from build123d import *

# Parameters (mm, degrees)
SKETCH1_W                    = 381
SKETCH1_H                    = 149.225
BOSS_EXTRUDE1_DEPTH          = 6.35
F_1_4_CLEARANCE_HOLE1_D      = 6.7564
CUT_EXTRUDE1_DEPTH           = 410.23028129
F_1_2_0_5_DIAMETER_HOLE1_D   = 12.7
F_10_0_1935_DIAMETER_HOLE1_D = 4.9149
SKETCH9_W                    = 19.05
SKETCH9_H                    = 14.2875
CUT_EXTRUDE2_DEPTH           = 410.23028129
FILLET1_R                    = 3.175


with BuildPart() as part:
    # Sketch1 → Boss-Extrude1 (new body)
    with BuildSketch(Plane(origin=(0, 0, 0), x_dir=(1, 0, 0), z_dir=(0, 1, 0))):
        with Locations((190.5, 74.6125)):
            Rectangle(SKETCH1_W, SKETCH1_H)
        with BuildLine():
            Line((342.9, 95.25), (342.9, 53.975))
            ThreePointArc((342.9, 53.975), (341.97006403, 51.72993597), (339.725, 50.8))
            Line((339.725, 50.8), (257.175, 50.8))
            ThreePointArc((257.175, 50.8), (254.92993597, 51.72993597), (254, 53.975))
            Line((254, 53.975), (254, 95.25))
            ThreePointArc((254, 95.25), (254.92993597, 97.49506403), (257.175, 98.425))
            Line((257.175, 98.425), (339.725, 98.425))
            ThreePointArc((339.725, 98.425), (341.97006403, 97.49506403), (342.9, 95.25))
        make_face(mode=Mode.SUBTRACT)
        with BuildLine():
            Line((41.275, 98.425), (123.825, 98.425))
            ThreePointArc((123.825, 98.425), (126.07006403, 97.49506403), (127, 95.25))
            Line((127, 95.25), (127, 53.975))
            ThreePointArc((127, 53.975), (126.07006403, 51.72993597), (123.825, 50.8))
            Line((123.825, 50.8), (41.275, 50.8))
            ThreePointArc((41.275, 50.8), (39.02993597, 51.72993597), (38.1, 53.975))
            Line((38.1, 53.975), (38.1, 95.25))
            ThreePointArc((38.1, 95.25), (39.02993597, 97.49506403), (41.275, 98.425))
        make_face(mode=Mode.SUBTRACT)
    extrude(amount=BOSS_EXTRUDE1_DEPTH)

    # 1/4 Clearance Hole1 (through all)
    with Locations(Plane(origin=(0, 6.35, 0), x_dir=(1, 0, 0), z_dir=(0, 1, 0))):
        with Locations((154.94, 74.6125), (186.69, 74.6125), (194.31, 74.6125), (226.06, 74.6125)):
            Hole(F_1_4_CLEARANCE_HOLE1_D / 2)

    # Sketch4 → Cut-Extrude1 (cut, through all)
    with BuildSketch(Plane(origin=(0, 6.35, 0), x_dir=(1, 0, 0), z_dir=(0, 1, 0))):
        with BuildLine():
            Line((186.69, 77.9907), (194.31, 77.9907))
            ThreePointArc((194.31, 77.9907), (197.6882, 74.6125), (194.31, 71.2343))
            Line((194.31, 71.2343), (186.69, 71.2343))
            ThreePointArc((186.69, 71.2343), (183.3118, 74.6125), (186.69, 77.9907))
        make_face()
    extrude(amount=-CUT_EXTRUDE1_DEPTH, mode=Mode.SUBTRACT)

    # 1/2 (0.5) Diameter Hole1 (through all)
    with Locations(Plane(origin=(19.05, 6.35, -130.175), x_dir=(0, 0, 1), z_dir=(0, 1, 0))):
        with Locations((0, 0), (111.125, 0), (0, 342.9), (111.125, 342.9)):
            Hole(F_1_2_0_5_DIAMETER_HOLE1_D / 2)

    # #10 (0.1935) Diameter Hole1 (through all)
    with Locations(Plane(origin=(0, 6.35, 0), x_dir=(1, 0, 0), z_dir=(0, 1, 0))):
        with Locations((19.05, 74.6125), (361.95, 74.6125)):
            Hole(F_10_0_1935_DIAMETER_HOLE1_D / 2)

    # Sketch9 → Cut-Extrude2 (cut, through all)
    with BuildSketch(Plane(origin=(0, 6.35, 0), x_dir=(1, 0, 0), z_dir=(0, 1, 0))):
        with Locations((117.475, 102.39375)):
            Rectangle(SKETCH9_W, SKETCH9_H)
        with Locations((117.475, 46.83125)):
            Rectangle(SKETCH9_W, SKETCH9_H)
        with Locations((263.525, 46.83125)):
            Rectangle(SKETCH9_W, SKETCH9_H)
        with Locations((263.525, 102.39375)):
            Rectangle(SKETCH9_W, SKETCH9_H)
    extrude(amount=-CUT_EXTRUDE2_DEPTH, mode=Mode.SUBTRACT)

    # Fillet1
    fillet1_edges = [part.edges().sort_by_distance(p)[0] for p in [
        (273.05, 3.175, -50.8),
        (273.05, 3.175, -98.425),
        (107.95, 3.175, -98.425),
        (107.95, 3.175, -50.8),
        (273.05, 3.175, -109.5375),
        (254, 3.175, -109.5375),
        (273.05, 3.175, -39.6875),
        (254, 3.175, -39.6875),
        (107.95, 3.175, -39.6875),
        (127, 3.175, -39.6875),
        (107.95, 3.175, -109.5375),
        (127, 3.175, -109.5375),
    ]]
    fillet(fillet1_edges, radius=FILLET1_R)


solid = part.part
The listing builds one solid part. Answer for the finished solid, in the listing's coordinates (mm). A direction names the side the tool comes from. Coordinates: 2 decimals unless noted, no trailing zeros. Loops run counter-clockwise (first coordinate to the right, second up) from the corner with the lowest first, then second, coordinate; pieces in that order, holes last. Notation, with made-up numbers: (9.5, -3) -> (41.5, -3) arc R11 cw to (41.5, 7) -> close; hole circle Ø2 at (33, 7). An arc over 180 degrees is marked (long way). Answer in a Markdown table with one row per item. Add a question column.
1. Consider line 1 (X direction, y = 4.5, z = -85.5); line 2 (Z direction, x = 361.95, y = 4.5) (3 decimals); line 3 (X direction, y = 3.5, z = -130). Determine where each line is inside the solid, lowest interval first. Write a range as [from, to].
2. A flat-ended cylindrical pin translates along its axis: P1, Ø1.9, axis at x = 190, y = 2.5, coming from the +Z side. Find the tip coordinate at first contact, or state that the pin passes through.
3. The part is cut by section C-C, the plane x = 68. Write down the section's boundary in (y, z) (3 decimals), then the cut area to 3 significant figures.
4. For faces 4 (the flat face through (73, 3, -98.425)), 5 (the flat face through (188, 3, 0)), determine the directions among +Z, -Z, +X, -X, +Y, -Y from which every point of the face is accessible in a straight line to the end or side of a thin tool.
5. The part is cut by section B-B, the plane x = 226.06. Write down the section's boundary in (y, z) (3 decimals), then the cut area to 3 significant figures.
6. The part is cut by section A-A, the plane z = -82.5. Write down the section's boundary in (x, y), then the cut area to 3 significant figures.
7. The part is cut by section D-D, the plane z = -129. Write down the section's boundary in (x, y), then the cut area to 3 significant figures.
8. Determine the mould class of faces 1 (the flat face through (73, 3, -50.8)), 2 (the flat face through (381, 3, -74)), 3 (the flat face through (188, 3, -149.225)) for opening direction X: +X half, -X half, draft (parallel to the pull), parting line (faces both ways), or undercut.
Answer below:
| question | item | result |
|---|---|---|
| 1 | line 1 | [0, 38.1], [127, 254], [342.9, 381] |
| 1 | line 2 | [-149.225, -136.525], [-123.825, -77.07], [-72.155, -25.4], [-12.7, 0] |
| 1 | line 3 | [0, 12.7], [25.4, 355.6], [368.3, 381] |
| 2 | P1 | z = 0 |
| 3 | outline | (0, -149.225) -> (6.35, -149.225) -> (6.35, -98.425) -> (0, -98.425) -> close; (0, -50.8) -> (6.35, -50.8) -> (6.35, 0) -> (0, 0) -> close |
| 3 | area | 645 mm2 |
| 4 | face 4 | +Y, -Y |
| 4 | face 5 | +Z, +X, -X, +Y, -Y |
| 5 | outline | (0, -149.225) -> (6.35, -149.225) -> (6.35, -77.991) -> (0, -77.991) -> close; (0, -71.234) -> (6.35, -71.234) -> (6.35, 0) -> (0, 0) -> close |
| 5 | area | 905 mm2 |
| 6 | outline | (0, 0) -> (38.1, 0) -> (38.1, 6.35) -> (0, 6.35) -> close; (127, 0) -> (254, 0) -> (254, 6.35) -> (127, 6.35) -> close; (342.9, 0) -> (381, 0) -> (381, 6.35) -> (342.9, 6.35) -> close |
| 6 | area | 1,290 mm2 |
| 7 | outline | (0, 0) -> (12.81, 0) -> (12.81, 6.35) -> (0, 6.35) -> close; (25.29, 0) -> (355.71, 0) -> (355.71, 6.35) -> (25.29, 6.35) -> close; (368.19, 0) -> (381, 0) -> (381, 6.35) -> (368.19, 6.35) -> close |
| 7 | area | 2,260 mm2 |
| 8 | face 1 | undercut |
| 8 | face 2 | +X half |
| 8 | face 3 | draft |
